Verification items for the finished model (mm, model axes). Give positions to 0.01 mm unless a question says otherwise; leave off trailing zeros. Loops run counter-clockwise (first coordinate to the right, second up) from the corner with the lowest first, then second, coordinate; pieces in that order, holes last. Notation, with made-up numbers: (46, 5) - (78, 5) arc R22 ccw to (78, 17) - close; hole circle Ø3 at (-35, 88.5). An arc over 180 degrees is marked (long way). Put each result on its own line as item: value. Start each with the question number.
```python
from build123d import *

# Parameters (mm, degrees)
F0_R     = 34.925
F0_R_2   = 25.4
F1_DEPTH = 85.344
F2_DEPTH = 76.2


with BuildPart() as f1:
    # F0 (on Front) → F1 (new body)
    with BuildSketch(Plane.XZ):
        Circle(F0_R)
        Circle(F0_R_2, mode=Mode.SUBTRACT)
    extrude(amount=F1_DEPTH)

    # F0 (on Front) → F2 (join)
    with BuildSketch(Plane.XZ):
        Polygon((38.1, 38.1), (0, 38.1), (-38.1, 38.1), (-38.1, -38.1), (38.1, -38.1), align=None)
        Circle(F0_R, mode=Mode.SUBTRACT)
    extrude(amount=F2_DEPTH)


solid = f1.part
```
1) Scan lines: line 1 along Z through (x, y) = (0, -24); line 2 along X through (y, z) = (-68.5, -17); line 3 along Y through (x, z) = (-29, -26). Record each from-to range of solid material in increasing order. Write a range as from..to.
2) Draft check along Z on faces 1 (the face through (-5.506, -42.075, -24.796)), 2 (the face through (-17, -76.2, -31)), 3 (the face through (-27.715, -80.708, -21.251)). Enter one of: pulls with the +Z half, pulls with the -Z half, needs draft (parallel to the pull), parting line crosses it, or undercut.
3) Section check A-A, the plane x = 0. Enter the section's corners in (y, z) (3 decimals), plus the area to 3 significant figures.
4) Section check B-B, the plane z = 0. Enter the section's corners in (x, y) (3 decimals).
5) Section check C-C, the plane y = -19.5. Enter the section's corners in (x, z), plus the area to 3 significant figures.
6) Section check D-D, the plane x = -29. Enter the section's corners in (y, z).
Results are:
1. line 1: z = -38.1..-25.4, 25.4..38.1
1. line 2: x = -38.1..-18.87, 18.87..38.1
1. line 3: y = -76.2..0
2. face 1: undercut
2. face 2: needs draft
2. face 3: parting line crosses it
3. outline: (-85.344, -34.925) - (-76.2, -34.925) - (-76.2, -38.1) - (0, -38.1) - (0, -25.4) - (-85.344, -25.4) - close; (-85.344, 25.4) - (0, 25.4) - (0, 38.1) - (-76.2, 38.1) - (-76.2, 34.925) - (-85.344, 34.925) - close
3. area: 2,110 mm2
4. outline: (-38.1, -76.2) - (-34.925, -76.2) - (-34.925, -85.344) - (-25.4, -85.344) - (-25.4, 0) - (-38.1, 0) - close; (25.4, -85.344) - (34.925, -85.344) - (34.925, -76.2) - (38.1, -76.2) - (38.1, 0) - (25.4, 0) - close
5. outline: (-38.1, -38.1) - (38.1, -38.1) - (38.1, 38.1) - (-38.1, 38.1) - close; hole circle Ø50.8 at (0, 0)
5. area: 3,780 mm2
6. outline: (-85.34, -19.46) - (-76.2, -19.46) - (-76.2, -38.1) - (0, -38.1) - (0, 38.1) - (-76.2, 38.1) - (-76.2, 19.46) - (-85.34, 19.46) - close
